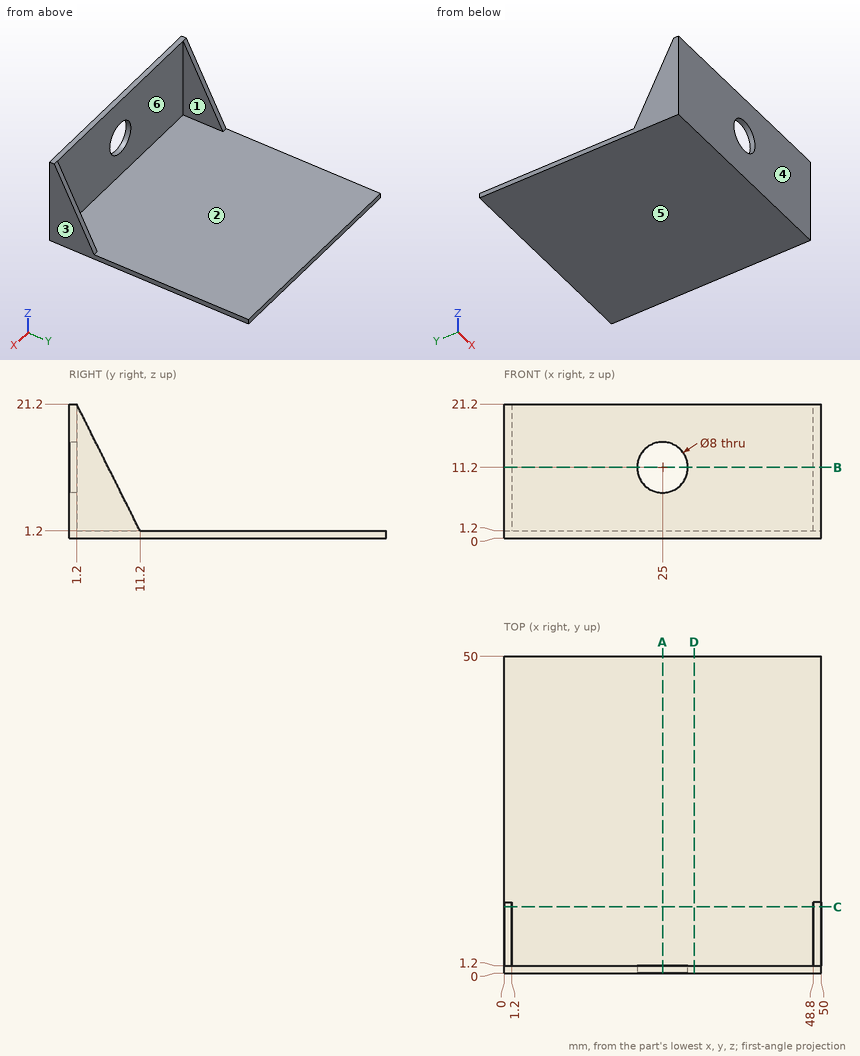
Could you check a few things on this drawing? It's one solid part, dimensions in mm from its lowest x, y, z. A direction names the side the tool comes from. Round coordinates to 2 decimals unless told otherwise and drop trailing zeros. Order: outer loops, then holes, each group sorted by start corner. A loop starts at its lowest first (then second) coordinate and runs counter-clockwise, first axis right, second up.
Q1. Please list where these lines run through material, in increasing order: probe 1 along Z at (x, y) = (25, 0.4); probe 2 along Z at (x, y) = (32, 35).
Geometry says:
probe 1: z = 0 to 7.2, 15.2 to 21.2
probe 2: z = 0 to 1.2
Q2. Imagine slicing it at B-B, the plane z = 11.2. List the corners of the cut face in (x, y) for me.
Geometry says:
outline: (0, 0) - (21, 0) - (21, 1.2) - (1.2, 1.2) - (1.2, 6.2) - (0, 6.2) - close; (29, 0) - (50, 0) - (50, 6.2) - (48.8, 6.2) - (48.8, 1.2) - (29, 1.2) - close
Q3. I'm going to push flat-ended pins straight in: P1, Ø10.5, axis at x = 25, z = 11.2, coming from the +Y side; P2, Ø1.5, axis at y = 5.5, z = 18, coming from the +X side; P3, Ø1.5, axis at x = 15, y = 7, coming from the +Z side. Where does each tip first touch, or does it pass through?
Geometry says:
P1: stops at y = 1.2
P2: passes through
P3: stops at z = 1.2
Q4. Imagine slicing it at A-A, the plane x = 25. List the corners of the cut face in (y, z) for me, then the cut area to 3 significant figures.
Geometry says:
outline: (0, 0) - (50, 0) - (50, 1.2) - (1.2, 1.2) - (1.2, 7.2) - (0, 7.2) - close; (0, 15.2) - (1.2, 15.2) - (1.2, 21.2) - (0, 21.2) - close
area: 74.4 mm2
Q5. Which directions (+Z, -Z, +X, -X, +Y, -Y) give clear straight access to the entire face, cutting with the end or side of a thin tool? Please do the marked faces 5 and 6.
Geometry says:
face 5: -Z, +X, -X, +Y, -Y
face 6: +Z, +Y
Q6. Imagine slicing it at D-D, the plane x = 30. List the corners of the cut face in (y, z) for me.
Geometry says:
outline: (0, 0) - (50, 0) - (50, 1.2) - (1.2, 1.2) - (1.2, 21.2) - (0, 21.2) - close
Q7. Thinking about a two-plate mould opening in X: for the marked faces 1, 2, 3 and 4, which applies, released by +X, released by -X, zero draft, split by the parting line, or undercut?
Geometry says:
face 1: undercut
face 2: undercut
face 3: released by +X
face 4: zero draft
Q8. Imagine slicing it at C-C, the plane y = 10.5. List the corners of the cut face in (x, z) for me, then the cut area to 3 significant figures.
Geometry says:
outline: (0, 0) - (50, 0) - (50, 2.6) - (48.8, 2.6) - (48.8, 1.2) - (1.2, 1.2) - (1.2, 2.6) - (0, 2.6) - close
area: 63.4 mm2
